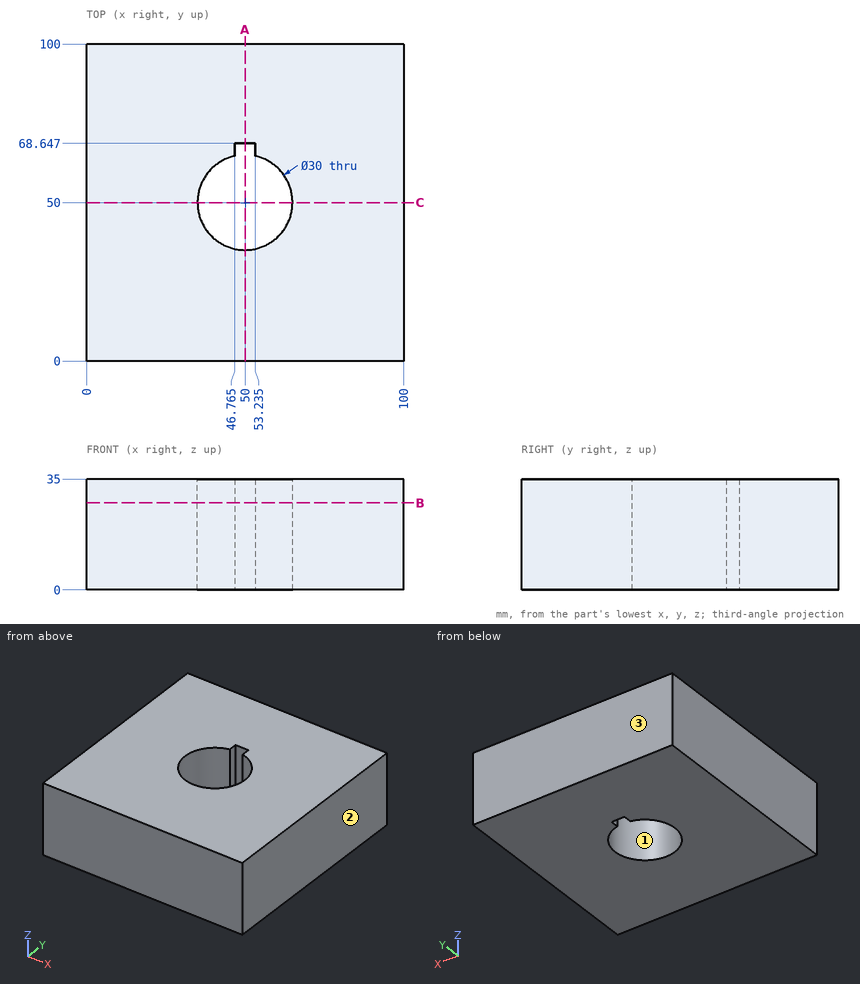
Design review of the part shown in the three views and the two pictorial views. Dimensions are in mm from the part's minimum x, y and z. Round coordinates to 2 decimals unless told otherwise and drop trailing zeros. Loops run counter-clockwise (first coordinate to the right, second up) from the corner with the lowest first, then second, coordinate; pieces in that order, holes last.
(1) Mouldability with a two-part tool opening along Y and no side actions: class the marked faces 1, 2 and 3 as released by +Y, released by -Y, zero draft, split by the parting line, or undercut.
Returned:
face 1: undercut
face 2: zero draft
face 3: released by +Y
(2) We need section B-B (z = 27.5). Give the boundary of the cut face in (x, y) (3 decimals).
Returned:
outline: (0, 0) - (100, 0) - (100, 100) - (0, 100) - close; hole (46.765, 64.647) arc R15 ccw (long way) to (53.235, 64.647) - (53.235, 68.647) - (46.765, 68.647) - close
(3) We need section C-C (y = 50). Give the boundary of the cut face in (x, z), plus the area to 3 significant figures.
Returned:
outline: (0, 0) - (35, 0) - (35, 35) - (0, 35) - close; (65, 0) - (100, 0) - (100, 35) - (65, 35) - close
area: 2,450 mm2
(4) Wall thickness on line 1 along X through (y, z) = (67, 6) (3 decimals); line 2 along X through (y, z) = (50, 23); line 3 along Y through (x, z) = (50, 7): over which ranges is each line inside the solid? List them lowest first.
Returned:
line 1: x = 0 to 46.765, 53.235 to 100
line 2: x = 0 to 35, 65 to 100
line 3: y = 0 to 35, 68.65 to 100
(5) We need section A-A (x = 50). Give the boundary of the cut face in (y, z).
Returned:
outline: (0, 0) - (35, 0) - (35, 35) - (0, 35) - close; (68.65, 0) - (100, 0) - (100, 35) - (68.65, 35) - close
